Geometry: final body of the model. Coordinates: model frame, mm. Face numbers are marked on the shaded views. A direction names the side the tool comes from. Give positions to 0.01 mm unless a question says otherwise; leave off trailing zeros. Order: outer loops, then holes, each group sorted by start corner. A loop starts at its lowest first (then second) coordinate and runs counter-clockwise, first axis right, second up. Notation, with made-up numbers: M -9,30 L 48,30 A20 cw 48,40 Z; hole C -25,45 d6. An arc over 180 degrees is marked long. Use CSV: the item, a comma, the result in double quotes.
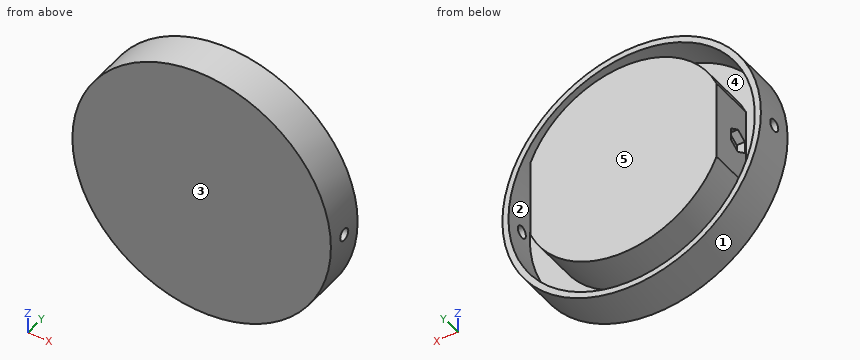
Autodesk Inventor part; units mm, degrees
ref_plane "Work Plane1" through (32, 0, 0) normal (1, 0, 0) x (0, 1, 0)
ref_plane "XZ Plane" through (0, 0, 0) normal (0, 1, 0) x (-1, 0, 0)
ref_plane "XY Plane" through (0, 0, 0) normal (0, 0, 1) x (1, 0, 0)
sketch "Sketch1" plane through (0, 0, 0) normal (0, 1, 0) x (-1, 0, 0)
  circle A0 centre (0, 0) radius 32
  dimension "d0" = 64
extrude "Extrusion1" add sketch "Sketch1" along normal blind 10
sketch "Sketch2" plane through (0, 10, 0) normal (0, 1, 0) x (1, 0, 0)
  circle A0 centre (0, 0) radius 30.5
  dimension "d3" = 61
extrude "Extrusion2" cut sketch "Sketch2" against normal blind 8
ref_plane "Work Plane1" through (32, 0, 0) normal (1, 0, 0) x (0, 1, 0)
sketch "Sketch5" plane through (32, 0, 0) normal (1, 0, 0) x (0, 1, 0)
  circle A0 centre (5, 0) radius 1.5
  line L0 (10, -32) -> (10, 32)
  point P0 (0, 0)
  dimension "d7" = 3
  dimension "d8" = 5
extrude "Extrusion3" cut sketch "Sketch5" against normal through all
sketch "Esquisse6" plane through (0, 2, 0) normal (0, 1, 0) x (1, 0, 0)
  circle A0 centre (0, 0) radius 25
  dimension "d11" = 50
extrude "Extrusion4" add sketch "Esquisse6" along normal blind 11
sketch "Esquisse7" plane through (0, 13, 0) normal (0, 1, 0) x (1, 0, 0)
  circle A0 centre (0, 0) radius 25
  line L0 (23, -9.798) -> (23, 9.798)
  line L1 (-23, -9.798) -> (-23, 9.798)
  dimension "d16" = 2
  dimension "d17" = 2
extrude "Extrusion5" cut sketch "Esquisse7" against normal blind 11 contours A0 L0 | L1 A0
sketch "Esquisse8" plane through (23, 13, 9.798) normal (1, 0, 0) x (0, 0, -1)
  line L0 (6.798, -8) -> (8.298, -5.4019)
  line L1 (8.298, -5.4019) -> (11.298, -5.4019)
  line L2 (11.298, -5.4019) -> (12.798, -8)
  line L3 (12.798, -8) -> (11.298, -10.5981)
  line L4 (11.298, -10.5981) -> (8.298, -10.5981)
  line L5 (8.298, -10.5981) -> (6.798, -8)
  line L6 (0, -11) -> (19.5959, -11)
  point P0 (9.798, -13)
  point P1 (11.298, -8)
  point P2 (9.798, -8)
  dimension "d18" = 6
extrude "Extrusion6" cut sketch "Esquisse8" against normal blind 2
sketch "Esquisse9" plane through (-23, 13, -9.798) normal (-1, 0, 0) x (0, 0, 1)
  line L0 (12.798, -8) -> (11.298, -10.5981)
  line L1 (11.298, -10.5981) -> (8.298, -10.5981)
  line L2 (8.298, -10.5981) -> (6.798, -8)
  line L3 (6.798, -8) -> (8.298, -5.4019)
  line L4 (8.298, -5.4019) -> (11.298, -5.4019)
  line L5 (11.298, -5.4019) -> (12.798, -8)
  line L6 (0, -11) -> (19.5959, -11)
  point P0 (9.798, -13)
  point P1 (8.298, -8)
  point P2 (9.798, -8)
  dimension "d21" = 6
extrude "Extrusion7" cut sketch "Esquisse9" against normal blind 2
properties part number "bouchon2"
1. Section D-D, the plane x = 28. Return the cut outline in (y, z), plus the area to 3 significant figures.
Answer:
outline,"M 0,-15.49 L 10,-15.49 L 10,-12.09 L 2,-12.09 L 2,12.09 L 10,12.09 L 10,15.49 L 0,15.49 Z"
area,"116 mm2"
2. Reachability of the marked faces 4 and 5 from +Z, -Z, +X, -X, +Y, -Y: full face, straight path, thin tool, end or side. Return the list, or none.
Answer:
face 4,"+Y"
face 5,"+Z, -Z, +X, -X, +Y"
3. Pull-direction query (Z, two-part tool) for the marked faces 1, 2 and 3; classes: +Z half, -Z half, draft (parallel to the pull), parting line (faces both ways), or undercut.
Answer:
face 1,"parting line"
face 2,"undercut"
face 3,"draft"
4. Line query: line 1 (X direction, y = 7.75, z = 0); line 2 (X direction, y = 7.5, z = 0); line 3 (Z direction, x = -17, y = 4.75). Output: solid intervals per line, ascending.
Answer:
line 1,"-32 to -30.5, -23 to 23, 30.5 to 32"
line 2,"-32 to -30.5, -21 to 21, 30.5 to 32"
line 3,"-27.11 to -25.32, -18.33 to 18.33, 25.32 to 27.11"
5. Pin query (flat end, axial travel): pin 1 Ø5 at (x, y) = (-5, 11.5) entering from -Z; pin 2 Ø2.5 at (y, z) = (5, 0) entering from -X; pin 3 Ø3 at (x, y) = (-12, 4) entering from -Z. Return the tip coordinate at first contact, or that it passes through.
Answer:
pin 1,"z = -31.86"
pin 2,"x = -21"
pin 3,"z = -30.23"
6. Section B-B, the plane z = -16. Return the cut outline in (x, y).
Answer:
outline,"M -27.71,0 L 27.71,0 L 27.71,10 L 25.97,10 L 25.97,2 L 19.21,2 L 19.21,13 L -19.21,13 L -19.21,2 L -25.97,2 L -25.97,10 L -27.71,10 Z"
7. Section A-A, the plane x = 0. Return the cut outline in (y, z), plus the area to 3 significant figures.
Answer:
outline,"M 0,-32 L 10,-32 L 10,-30.5 L 2,-30.5 L 2,-25 L 13,-25 L 13,25 L 2,25 L 2,30.5 L 10,30.5 L 10,32 L 0,32 Z"
area,"702 mm2"
8. Section C-C, the plane y = 1.25. Return the cut outline in (x, z).
Answer:
outline,"C 0,0 d64"
